Work out the finished part from the listing and answer in its coordinate system (mm). Face numbers are marked on the shaded views. Give positions to 0.01 mm unless a question says otherwise; leave off trailing zeros. Order: outer loops, then holes, each group sorted by start corner. A loop starts at its lowest first (then second) coordinate and runs counter-clockwise, first axis right, second up. Notation, with made-up numbers: (50, 84) - (62, 84) arc R9 cw to (62, 90) - close; hole circle Ø6 at (-21, -3). An arc over 180 degrees is marked (long way). Put each result on its own line as item: value.
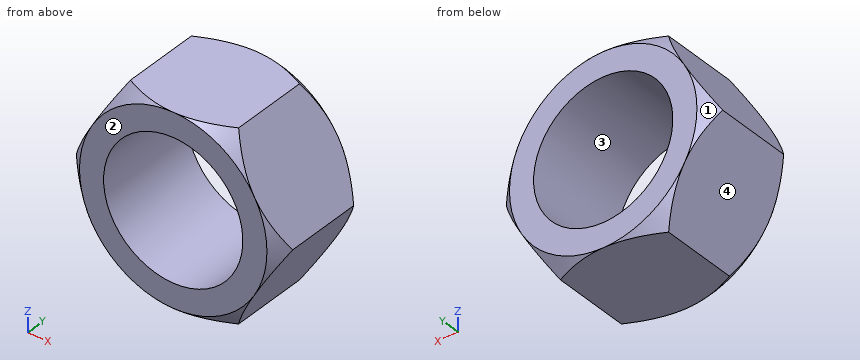
```python
from build123d import *

# Parameters (mm, degrees)
SKETCH1_R           = 3.302
BOSS_EXTRUDE1_DEPTH = 2.54


# Read off the part's stored shape, not the designer's step: Cut-Extrude1
with BuildPart() as part:
    # Sketch1 → Boss-Extrude1 (new, symmetric)
    with BuildSketch(Plane(origin=(0, 0, 0), x_dir=(1, 0, 0), z_dir=(0, 1, 0))):
        Polygon((5.132643893, 0), (2.566321947, 4.445), (-2.566321947, 4.445), (-5.132643893, 0), (-2.566321947, -4.445), (2.566321947, -4.445), align=None)
        with Locations(Location((0, 0, 0), (0, 0, 270))):
            Circle(SKETCH1_R, mode=Mode.SUBTRACT)
    extrude(amount=BOSS_EXTRUDE1_DEPTH, both=True)

    # Cut-Extrude1 outline → Cut-Extrude1 (revolve, cut)
    with BuildSketch(Plane.XY):
        Polygon((5.132643901, 2.540000192), (4.444999936, 2.540000192), (5.132643898, 1.852356102), align=None)
    cut_extrude1 = revolve(axis=Axis((0, 0, 0), (0, 1, 0)), mode=Mode.SUBTRACT)

    # Mirror1: Cut-Extrude1 across plane
    add(cut_extrude1.mirror(Plane.ZX), mode=Mode.SUBTRACT)


solid = part.part
```
(1) Section B-B, the plane y = 2.25 is taken. Write down the section's boundary in (x, z) (3 decimals).
Geometry check:
outline: (-4.665, -0.809) - (-3.034, -3.636) arc R4.735 ccw to (-1.632, -4.445) - (1.632, -4.445) arc R4.735 ccw to (3.034, -3.636) - (4.665, -0.809) arc R4.735 ccw to (4.665, 0.809) - (3.034, 3.636) arc R4.735 ccw to (1.632, 4.445) - (-1.632, 4.445) arc R4.735 ccw to (-3.034, 3.636) - (-4.665, 0.809) arc R4.735 ccw to start; hole circle Ø6.604 at (0, 0)
(2) Section A-A, the plane y = -0.3 is taken. Write down the section's boundary in (x, z) (3 decimals), then the cut area to 3 significant figures.
Geometry check:
outline: (-5.133, 0) - (-2.566, -4.445) - (2.566, -4.445) - (5.133, 0) - (2.566, 4.445) - (-2.566, 4.445) - close; hole circle Ø6.604 at (0, 0)
area: 34.2 mm²
(3) Determine the mould class of the marked faces 1, 2, 3 and 4 for opening direction Z: pulls with the +Z half, pulls with the -Z half, needs draft (parallel to the pull), parting line crosses it, or undercut.
Geometry check:
face 1: parting line crosses it
face 2: needs draft
face 3: undercut
face 4: pulls with the -Z half
(4) Given pin 1 (4 mm diameter, centred on x = 1, z = 0, fed in from -Y), flat-ended and moving along its own axis, determine where the tip first touches the part or whether it passes through.
Geometry check:
pin 1: passes through
(5) Straight lines are drawn through the part: line 1 (X direction, y = -1, z = -1.75); line 2 (X direction, y = 1.4, z = 0.25); line 3 (Z direction, x = 3, y = -0.4). For each, find the intervals that lie inside material, in ascending order.
Geometry check:
line 1: x = -4.12 to -2.8, 2.8 to 4.12
line 2: x = -4.99 to -3.29, 3.29 to 4.99
line 3: z = -3.69 to -1.38, 1.38 to 3.69
